Check sheet for the drawn part. Datum: minimum x, y, z corner. Units: mm. Give positions to 0.01 mm unless a question says otherwise; leave off trailing zeros. Write each loop counter-clockwise with the first axis right and the second up, starting at its lowest first coordinate (ties: lowest second). Pieces come first, ordered by that corner, then holes. Notation, with made-up numbers: (35.5, 46.5) - (87.5, 46.5) arc R18 ccw to (87.5, 69.5) - close; hole circle Ø7 at (3.25, -33). An arc over 180 degrees is marked (long way). One line per question, with ' | ' between items. Start each with the question number.
Q1. Section check A-A on x = 160. Record the boundary of the cut face in (y, z).
Q2. Thickness scan on L1, parallel to X at y = 6.5, z = 21; L2, parallel to Z at x = 160, y = 7; L3, parallel to X at y = 7, z = 18.5. Record the ranges inside material, lowest first. Write a range as [from, to].
Q3. Section check C-C on y = 5.75. Record the boundary of the cut face in (x, z), and give its area (3 significant figures).
Q4. Section check B-B on z = 21. Record the boundary of the cut face in (x, y).
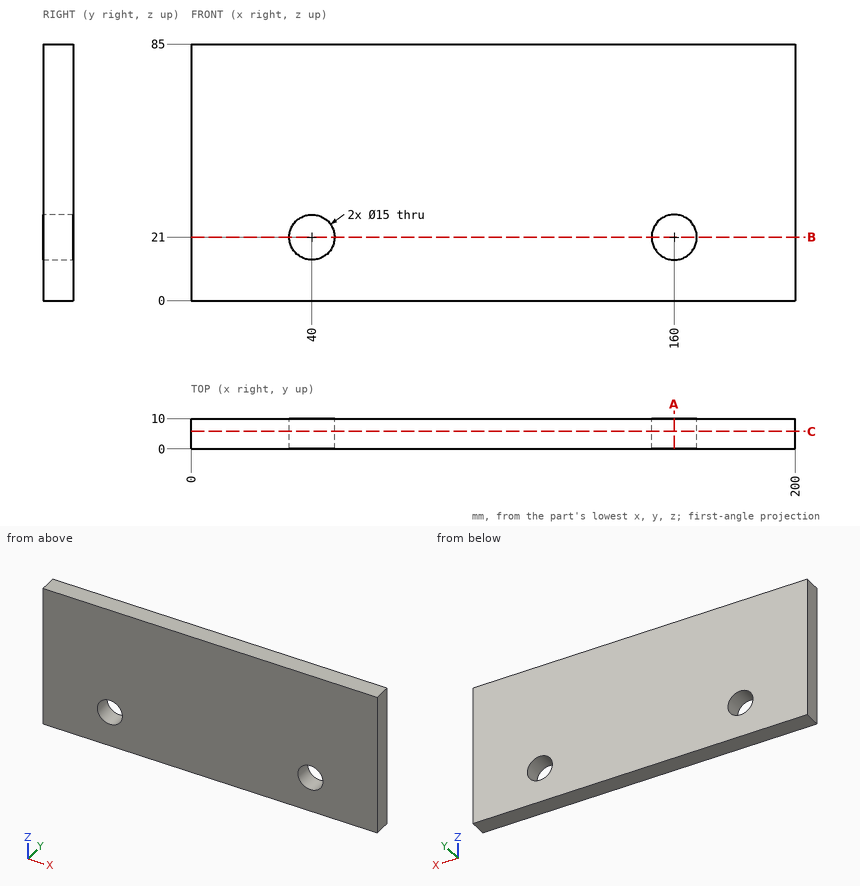
Working result:
1) outline: (0, 0) - (10, 0) - (10, 13.5) - (0, 13.5) - close; (0, 28.5) - (10, 28.5) - (10, 85) - (0, 85) - close
2) L1: x = [0, 32.5], [47.5, 152.5], [167.5, 200] | L2: z = [0, 13.5], [28.5, 85] | L3: x = [0, 32.93], [47.07, 152.93], [167.07, 200]
3) outline: (0, 0) - (200, 0) - (200, 85) - (0, 85) - close; hole circle Ø15 at (40, 21); hole circle Ø15 at (160, 21) | area: 16,600 mm2
4) outline: (0, 0) - (32.5, 0) - (32.5, 10) - (0, 10) - close; (47.5, 0) - (152.5, 0) - (152.5, 10) - (47.5, 10) - close; (167.5, 0) - (200, 0) - (200, 10) - (167.5, 10) - close
